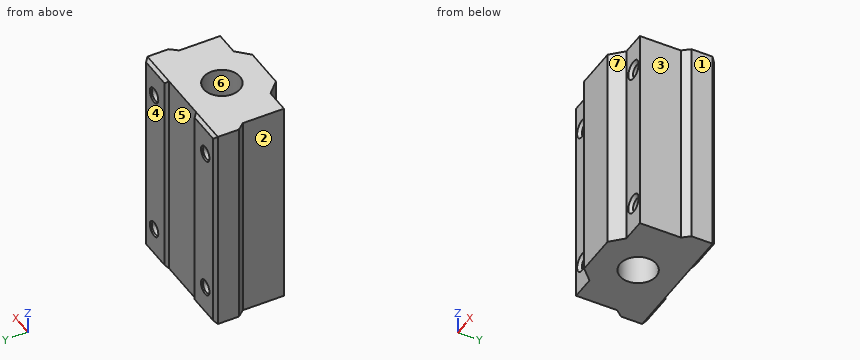
```python
from build123d import *

# Parameters (mm, degrees)
ESBO_O1_R                       = 6
RESSALTO_EXTRUS_O1_DEPTH        = 70
CHANFRO1_SIZE                   = 1
FURO_ROSCADO_DE_M51_D           = 4.2
FURO_ROSCADO_DE_M51_CSINK_D     = 5.05
FURO_ROSCADO_DE_M51_CSINK_ANGLE = 90
CHANFRO2_SIZE                   = 1


with BuildPart() as part:
    # Esboço1 → Ressalto-extrusão1 (new body)
    with BuildSketch(Plane.XY):
        Polygon((8, 13), (-8, 13), (-8, 14), (-21, 14), (-21, 6), (-19, 3.616492815), (-19, -10), (-11, -10), (-7, -14), (7, -14), (11, -10), (19, -10), (19, 3.616492815), (21, 6), (21, 14), (8, 14), align=None)
        Circle(ESBO_O1_R, mode=Mode.SUBTRACT)
    extrude(amount=-RESSALTO_EXTRUS_O1_DEPTH)

    # Chanfro1
    chanfro1_edges = [part.edges().sort_by_distance(p)[0] for p in [
        (14.5, 14, -70),
        (21, 14, -35),
        (14.5, 14, 0),
        (8, 14, -35),
        (-14.5, 14, -70),
        (-21, 14, -35),
        (-14.5, 14, 0),
        (-8, 14, -35),
    ]]
    chamfer(chanfro1_edges, length=CHANFRO1_SIZE - 0.0001)  # a hair under: the kernel refuses the full size

    # Furo roscado de M51 (through all)
    with Locations(Plane(origin=(0, 14, 0), x_dir=(1, 0, 0), z_dir=(0, 1, 0))):
        with Locations((15.25, 10), (15.25, 60), (-15.25, 60), (-15.25, 10)):
            CounterSinkHole(FURO_ROSCADO_DE_M51_D / 2, FURO_ROSCADO_DE_M51_CSINK_D / 2, counter_sink_angle=FURO_ROSCADO_DE_M51_CSINK_ANGLE)

    # Chanfro2
    chanfro2_edges = [part.edges().sort_by_distance(p)[0] for p in [
        (-13.15, -10, -10),
        (-13.15, -10, -60),
        (17.35, -10, -60),
        (17.35, -10, -10),
    ]]
    chamfer(chanfro2_edges, length=CHANFRO2_SIZE)


solid = part.part
```
Design review of the part built by this model. Coordinates are the model's own, in mm. Face numbers are marked on the shaded views. A direction names the side the tool comes from. Coordinates: 2 decimals unless noted, no trailing zeros. Order: outer loops, then holes, each group sorted by start corner. A loop starts at its lowest first (then second) coordinate and runs counter-clockwise, first axis right, second up. Notation, with made-up numbers: (47.5, 60) -> (83.5, 60) arc R31 ccw to (83.5, 93) -> close; hole circle Ø4 at (-18.75, 30). An arc over 180 degrees is marked (long way). One line per item, written item: value. Start each with the question number.
Q1. Tool access review of the marked faces 1, 2 and 3: name each direction out of +Z, -Z, +X, -X, +Y, -Y from which nothing blocks a thin tool from reaching the whole face with its end or side.
Q2. Insertion check: pin 1 Ø15 at (y, z) = (-5, -39.5) entering from -X; pin 2 Ø7 at (y, z) = (-6.5, -40) entering from +X; pin 3 Ø4 at (x, z) = (3, -25.5) entering from +Y; pin 4 Ø3.5 at (x, z) = (-15.25, -60) entering from +Y. Each pin has a flat end and moves straight along its axis. Give the tip position at first contact, or say it passes through.
Q3. Take a section at B-B, the plane x = 0. State the section outline as (y, z) points, then the cut area to 3 significant figures.
Q4. For probe 1 along X at (y, z) = (8, -60); probe 2 along Z at (x, y) = (15.25, 5.5); probe 3 along Y at (x, z) = (0, -52), list the stretches that pass through material, from the lowest coordinate up.
Q5. Mouldability with a two-part tool opening along X and no side actions: class the marked faces 4, 5, 6 and 7 as pulls with the +X half, pulls with the -X half, needs draft (parallel to the pull), parting line crosses it, or undercut.
Q6. Take a section at D-D, the plane z = -60. Give the number of separate pieces and of enclosed holes in the cut face, then the cut area to 3 significant figures.
Q7. Take a section at A-A, the plane y = 0. State the section outline as (x, z) points, then the cut area to 3 significant figures.
Values follow:
1. face 1: +Z, -Z, +X, +Y, -Y
1. face 2: +Z, -Z, -X, -Y
1. face 3: +Z, -Z, +X, -Y
2. pin 1: stops at x = -19
2. pin 2: stops at x = 19
2. pin 3: stops at y = 13
2. pin 4: passes through
3. outline: (-14, -70) -> (-6, -70) -> (-6, 0) -> (-14, 0) -> close; (6, -70) -> (13, -70) -> (13, 0) -> (6, 0) -> close
3. area: 1,050 mm2
4. probe 1: x = -21 to -17.35, -13.15 to 13.15, 17.35 to 21
4. probe 2: z = -70 to -62.1, -57.9 to -12.1, -7.9 to 0
4. probe 3: y = -14 to -6, 6 to 13
5. face 4: needs draft
5. face 5: undercut
5. face 6: undercut
5. face 7: pulls with the +X half
6. separate pieces: 3
6. enclosed holes: 1
6. area: 686 mm2
7. outline: (-19, -70) -> (-6, -70) -> (-6, 0) -> (-19, 0) -> close; (6, -70) -> (19, -70) -> (19, 0) -> (6, 0) -> close; hole circle Ø4.2 at (-15.25, -60); hole circle Ø4.2 at (-15.25, -10); hole circle Ø4.2 at (15.25, -60); hole circle Ø4.2 at (15.25, -10)
7. area: 1,760 mm2
